Here's how the part is built. I have some questions about the finished solid (model axes, mm). A direction names the side the tool comes from. Give positions to 0.01 mm unless a question says otherwise; leave off trailing zeros. Order: outer loops, then holes, each group sorted by start corner. A loop starts at its lowest first (then second) coordinate and runs counter-clockwise, first axis right, second up. Notation, with made-up numbers: (86.25, -34.5) -> (144.25, -34.5) arc R10 ccw to (144.25, -22.5) -> close; hole circle Ø2 at (-23.5, -5). An arc over 180 degrees is marked (long way). Write each question's results on one line, items separated by ' | '. Start each with the question number.
Q1. I need wall thicknesses on line 1 along Y through (x, z) = (2.75, 1.9); line 2 along X through (y, z) = (-0.35, 1.35); line 3 along X through (y, z) = (0.05, 1.35). Which ranges of each line are inside material? Lowest first, please. Write a range as [from, to].
Q2. I'm going to push flat-ended pins straight in: pin 1 (0.6 mm diameter, centred on y = 0.5, z = 1.5, fed in from -X); pin 2 (1 mm diameter, centred on x = 2, z = 0.5, fed in from -Y); pin 3 (0.6 mm diameter, centred on x = -1, z = 1.5, fed in from +Y). Where does each tip first touch, or does it pass through?
Q3. Imagine slicing it at C-C, the plane y = -0.65. Please give me the cut outline in (x, z), then the cut area to 3 significant figures.
Q4. Thinking about a two-plate mould opening in X: for faces 4 (the face through (-2, -1, 1)), 5 (the face through (3, 0.5, 1)), 6 (the face through (3, 0.3, 1)), which applies, pulls with the +X half, pulls with the -X half, needs draft (parallel to the pull), parting line crosses it, or undercut?
Q5. Imagine slicing it at A-A, the plane z = 1.1. Please give me the cut outline in (x, y).
Q6. For faces 1 (the face through (9, 0.3, 1)), 2 (the face through (-1, 0, 1)), 3 (the face through (7.01, -0.25, 0.99)), which set-ups out of +Z, -Z, +X, -X, +Y, -Y let a thin tool reach every point of the face, with its end or its side?
Q7. Imagine slicing it at B-B, the plane x = 4.5. Please give me the cut outline in (y, z), then the cut area to 3 significant figures.
```python
from build123d import *

# Parameters (mm, degrees)
EXTRUDE_1_DEPTH     = 2
SKETCH_3_W          = 0.25
SKETCH_3_H          = 1.3
CUT_EXTRUDE_2_DEPTH = 1.2


with BuildPart() as part:
    # 草图1 → 凸台-拉伸1 (new body)
    with BuildSketch(Plane.XY):
        with BuildLine():
            Line((0, 0), (0, 0.5))
            Line((0, 0.5), (6.45, 0.5))
            ThreePointArc((6.45, 0.5), (7, -0.05), (7.55, 0.5))
            Line((7.55, 0.5), (9.5, 0.5))
            Line((9.5, 0.5), (9.5, 0.3))
            Line((9.5, 0.3), (7.722841615, 0.3))
            ThreePointArc((7.722841615, 0.3), (7, -0.25), (6.277158385, 0.3))
            Line((6.277158385, 0.3), (0.2, 0.3))
            Line((0.2, 0.3), (0.2, -0.2))
            Line((0.2, -0.2), (-1.8, -0.2))
            Line((-1.8, -0.2), (-1.8, -1.5))
            Line((-1.8, -1.5), (-2, -1.5))
            Line((-2, -1.5), (-2, 0))
            Line((-2, 0), (0, 0))
        make_face()
    extrude(amount=EXTRUDE_1_DEPTH)

    # 草图3 → 切除-拉伸2 (cut, through all)
    with BuildSketch(Plane(origin=(-1.8, 0, 0), x_dir=(0, 0, -1), z_dir=(1, 0, 0))):
        with Locations((-1.875, -0.85)):
            Rectangle(SKETCH_3_W, SKETCH_3_H)
        with Locations((-0.125, -0.85)):
            Rectangle(SKETCH_3_W, SKETCH_3_H)
    extrude(amount=-CUT_EXTRUDE_2_DEPTH, mode=Mode.SUBTRACT)


solid = part.part
```
Geometry check:
1) line 1: [0.3, 0.5] | line 2: [-2, -1.8] | line 3: [0, 0.2], [6.4, 6.68], [7.32, 7.6]
2) pin 1: x = 0 | pin 2: y = 0.3 | pin 3: y = 0
3) outline: (-2, 0.25) -> (-1.8, 0.25) -> (-1.8, 1.75) -> (-2, 1.75) -> close | area: 0.300 mm²
4) face 4: pulls with the -X half | face 5: needs draft | face 6: undercut
5) outline: (-2, -1.5) -> (-1.8, -1.5) -> (-1.8, -0.2) -> (0.2, -0.2) -> (0.2, 0.3) -> (6.28, 0.3) arc R0.75 ccw to (7.72, 0.3) -> (9.5, 0.3) -> (9.5, 0.5) -> (7.55, 0.5) arc R0.55 cw to (6.45, 0.5) -> (0, 0.5) -> (0, 0) -> (-2, 0) -> close
6) face 1: +Z, -Z, +X, -Y | face 2: +Z, -Z, -X, +Y | face 3: +Z, -Z, -Y
7) outline: (0.3, 0) -> (0.5, 0) -> (0.5, 2) -> (0.3, 2) -> close | area: 0.400 mm²
